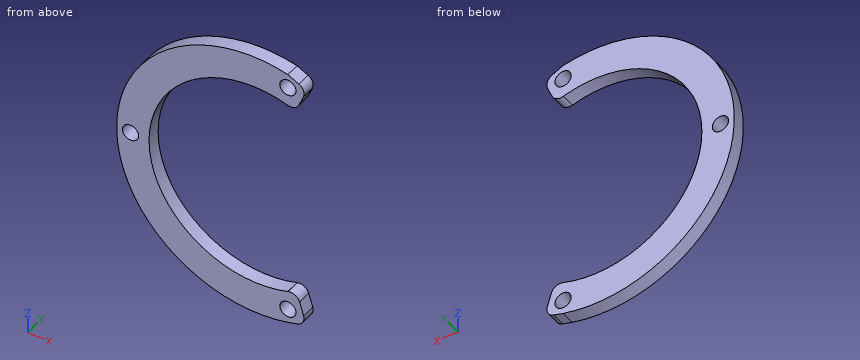
Autodesk Inventor part; units mm, degrees
ref_plane "YZ Plane" through (0, 0, 0) normal (1, 0, 0) x (0, 1, 0)
ref_plane "XZ Plane" through (0, 0, 0) normal (0, 1, 0) x (-1, 0, 0)
ref_plane "XY Plane" through (0, 0, 0) normal (0, 0, 1) x (1, 0, 0)
sketch "Sketch1" plane through (0, 0, 0) normal (0, 1, 0) x (-1, 0, 0)
  arc A0 (-7.2165, -28.9468) -> (-7.2165, 29.397) centre (-0.2165, 0.2251) ccw
  arc A1 (-7.2165, -25.8517) -> (-7.2165, 26.3019) centre (-0.2165, 0.2251) ccw construction
  arc A2 (-7.2165, -21.6838) -> (-7.2165, 22.134) centre (-0.2165, 0.2251) ccw
  line L0 (-7.2165, 33.9307) -> (-7.2165, -32.8883) construction
  circle A3 centre (-7.2165, 26.3019) radius 1.75
  circle A4 centre (-7.2165, -25.8517) radius 1.75
  circle A5 centre (26.7835, 0.2251) radius 1.75
  line L1 (-7.2165, 29.397) -> (-11.2926, 27.3801)
  line L2 (-11.2926, 27.3801) -> (-8.8324, 21.4622)
  line L3 (-8.8324, 21.4622) -> (-7.2165, 22.134)
  line L4 (-7.2165, -28.9468) -> (-11.2102, -27.8268)
  line L5 (-11.2102, -27.8268) -> (-9.1721, -21.092)
  line L6 (-9.1721, -21.092) -> (-7.2165, -21.6838)
  dimension "d14" = 54
  dimension "d16" = 46
  dimension "d17" = 30
  dimension "d19" = 3.5
  dimension "d20" = 3.5
  dimension "d21" = 7
  dimension "d22" = 3.5
extrude "Extrusion1" add sketch "Sketch1" along normal blind 3
fillet "Fillet1" radius 2 4 edges at (11.2926, 1.5, 27.3801) (8.8324, 1.5, 21.4622) (11.2102, 1.5, -27.8268) (9.1721, 1.5, -21.092)
properties part number "reverse gear reverse lever ring"
Can you work these out from the model? Positions are in its coordinate system, mm. Coordinates: 2 decimals unless noted, no trailing zeros. Order: outer loops, then holes, each group sorted by start corner. A loop starts at its lowest first (then second) coordinate and runs counter-clockwise, first axis right, second up.
1. If we section it at B-B (x = -20): Please give me the cut outline in (y, z).
2. If we section it at A-A (x = 6.5): Please give me the cut outline in (y, z).
3. If we section it at C-C (x = -5.5): Please give me the cut outline in (y, z).
4. I'm going to push a flat-ended pin straight in: pin 1 (1 mm diameter, centred on x = -13.5, y = 1.5, fed in from +Z). Where does the tip first touch, or does it pass through?
5. If we section it at D-D (z = -2.5): Please give me the cut outline in (x, y).
6. I need wall thicknesses on line 1 (Z direction, x = 1, y = 2.85); line 2 (Z direction, x = 3, y = 1.75); line 3 (X direction, y = 1.2, z = 4). Which ranges of each line are inside material? Lowest first, please.
Entries:
1. outline: (0, -21.94) - (3, -21.94) - (3, -10.74) - (0, -10.74) - close; (0, 11.19) - (3, 11.19) - (3, 22.39) - (0, 22.39) - close
2. outline: (0, -29.11) - (3, -29.11) - (3, -27.45) - (0, -27.45) - close; (0, -24.26) - (3, -24.26) - (3, -21.9) - (0, -21.9) - close; (0, 22.35) - (3, 22.35) - (3, 24.71) - (0, 24.71) - close; (0, 27.9) - (3, 27.9) - (3, 29.56) - (0, 29.56) - close
3. outline: (0, -29.23) - (3, -29.23) - (3, -22.05) - (0, -22.05) - close; (0, 22.5) - (3, 22.5) - (3, 29.68) - (0, 29.68) - close
4. pin 1: stops at z = 27.16
5. outline: (-29.66, 0) - (-22.62, 0) - (-22.62, 3) - (-29.66, 3) - close
6. line 1: z = -29.76 to -22.76, 23.21 to 30.21
6. line 2: z = -29.65 to -22.61, 23.06 to 30.1
6. line 3: x = -29.55 to -22.47
